Input: part model. Units: mm. Frame: model coordinates. A direction names the side the tool comes from. Give positions to 0.01 mm unless a question says otherwise; leave off trailing zeros. Order: outer loops, then holes, each group sorted by start corner. A loop starts at its lowest first (then second) coordinate and runs counter-clockwise, first axis right, second up. Notation, with made-up numbers: M 34.5,-34.5 L 78.5,-34.5 A22 ccw 78.5,0.5 Z; hole C 39.25,-28 d11. An arc over 180 degrees is marked long. Use a Markdown table: item, result.
from build123d import *

# Parameters (mm, degrees)
EXTRUDE_1_DEPTH     = 4
SKETCH_3_R          = 2
CUT_EXTRUDE_1_DEPTH = 272.02260581
SKETCH_4_R          = 10.5
SKETCH_4_R_2        = 1.5
CUT_EXTRUDE_2_DEPTH = 272.02260581
SKETCH_5_R          = 2
CUT_EXTRUDE_3_DEPTH = 272.02260581
SKETCH_6_W          = 10
SKETCH_6_H          = 62
CUT_EXTRUDE_4_DEPTH = 272.02260581
FILLET_1_R          = 10
SKETCH_7_W          = 13
SKETCH_7_H          = 13
CUT_EXTRUDE_5_DEPTH = 4
EXTRUDE_2_DEPTH     = 4
FILLET_2_R          = 10


with BuildPart() as part:
    # 草图2 → 凸台-拉伸1 (new body)
    with BuildSketch(Plane.XY):
        Polygon((0, 0), (-75, 0), (-75, -15), (-244.434557418, -15), (-55, -117), (0, -117), align=None)
    extrude(amount=EXTRUDE_1_DEPTH)

    # 草图3 → 切除-拉伸1 (cut, through all)
    with BuildSketch(Plane.XY.offset(4)):
        with Locations((-57.5, -6)):
            Circle(SKETCH_3_R)
        with Locations((-69, -17.5)):
            Circle(SKETCH_3_R)
        with Locations((-17.5, -6)):
            Circle(SKETCH_3_R)
        with Locations((-6, -17.5)):
            Circle(SKETCH_3_R)
        with Locations((-6, -57.5)):
            Circle(SKETCH_3_R)
        with Locations((-17.5, -69)):
            Circle(SKETCH_3_R)
        with Locations((-57.5, -69)):
            Circle(SKETCH_3_R)
        with Locations((-69, -57.5)):
            Circle(SKETCH_3_R)
    extrude(amount=-CUT_EXTRUDE_1_DEPTH, mode=Mode.SUBTRACT)

    # 草图4 → 切除-拉伸2 (cut, through all)
    with BuildSketch(Plane.XY.offset(4)):
        with Locations((-40, -100)):
            Circle(SKETCH_4_R)
        with Locations((-52.5, -112.5)):
            Circle(SKETCH_4_R_2)
        with Locations((-27.5, -112.5)):
            Circle(SKETCH_4_R_2)
        with Locations((-27.5, -87.5)):
            Circle(SKETCH_4_R_2)
        with Locations((-52.5, -87.5)):
            Circle(SKETCH_4_R_2)
    extrude(amount=-CUT_EXTRUDE_2_DEPTH, mode=Mode.SUBTRACT)

    # 草图5 → 切除-拉伸3 (cut, through all)
    with BuildSketch(Plane.XY.offset(4)):
        with Locations((-98.653292605, -71.825698472)):
            Circle(SKETCH_5_R)
        with Locations((-72.238972, -86.048344744)):
            Circle(SKETCH_5_R)
        with Locations((-160.286707351, -38.639523839)):
            Circle(SKETCH_5_R)
        with Locations((-186.701027956, -24.416877568)):
            Circle(SKETCH_5_R)
    extrude(amount=-CUT_EXTRUDE_3_DEPTH, mode=Mode.SUBTRACT)

    # 草图6 → 切除-拉伸4 (cut, through all)
    with BuildSketch(Plane.XY.offset(4)):
        with Locations((-5, -86)):
            Rectangle(SKETCH_6_W, SKETCH_6_H)
    extrude(amount=-CUT_EXTRUDE_4_DEPTH, mode=Mode.SUBTRACT)

    # 圆角1
    fillet_1_edges = [part.edges().sort_by_distance(p)[0] for p in [
        (0, -55, 2),
    ]]
    fillet(fillet_1_edges, radius=FILLET_1_R - 0.0001)  # a hair under: the kernel refuses the full size

    # 草图7 → 切除-拉伸5 (cut)
    with BuildSketch(Plane.XY.offset(4)):
        Polygon((-19.242640687, -15), (-55.757359313, -15), (-51.757359313, -19), (-23.242640687, -19), align=None)
        Polygon((-56, -23.242640687), (-60, -19.242640687), (-60, -55.757359313), (-56, -51.757359313), align=None)
        Polygon((-51.757359313, -56), (-55.757359313, -60), (-19.242640687, -60), (-23.242640687, -56), align=None)
        Polygon((-15, -55.757359313), (-15, -19.242640687), (-19, -23.242640687), (-19, -51.757359313), align=None)
        Polygon((-27.242640687, -23), (-47.757359313, -23), (-43.757359313, -27), (-31.242640687, -27), align=None)
        Polygon((-48, -31.242640687), (-52, -27.242640687), (-52, -47.757359313), (-48, -43.757359313), align=None)
        Polygon((-43.757359313, -48), (-47.757359313, -52), (-27.242640687, -52), (-31.242640687, -48), align=None)
        Polygon((-23, -47.757359313), (-23, -27.242640687), (-27, -31.242640687), (-27, -43.757359313), align=None)
        with Locations((-37.5, -37.5)):
            Rectangle(SKETCH_7_W, SKETCH_7_H)
    extrude(amount=-CUT_EXTRUDE_5_DEPTH, mode=Mode.SUBTRACT)

    # 草图8 → 凸台-拉伸2 (add)
    with BuildSketch(Plane.XY.offset(4)):
        with BuildLine():
            Line((-10, -117), (-55, -117))
            ThreePointArc((-55, -117), (-32.5, -122.672487724), (-10, -117))
        make_face()
    extrude(amount=-EXTRUDE_2_DEPTH)

    # 圆角2
    fillet_2_edges = [part.edges().sort_by_distance(p)[0] for p in [
        (-10, -117, 2),
        (-10, -55, 2),
        (-244.434557418, -15, 2),
        (-75, -15, 2),
    ]]
    fillet(fillet_2_edges, radius=FILLET_2_R)


solid = part.part
1) Reachability of faces 1 (the face through (-37, -56, 2)), 2 (the face through (-144, -15, 2)) from +Z, -Z, +X, -X, +Y, -Y: full face, straight path, thin tool, end or side. Return the list, or none.
Response values:
| item | result |
|---|---|
| face 1 | +Z, -Z |
| face 2 | +Z, -Z, -X, +Y |
2) First-contact query: pin 1 Ø5 at (x, y) = (-17.5, -6) entering from -Z; pin 2 Ø2 at (x, z) = (-37.5, 1) entering from -Y; pin 3 Ø1 at (x, z) = (-146.5, 3.5) entering from -Y; pin 4 Ø1.5 at (x, z) = (-133, 3.5) entering from -Y. Flat tips, straight axial feed; report the tip coordinate or a pass-through.
Response values:
| item | result |
|---|---|
| pin 1 | stops at z = 0 |
| pin 2 | stops at y = -122.5 |
| pin 3 | stops at y = -68 |
| pin 4 | stops at y = -75.41 |
3) Cut plane A-A on y = -100. Return loops of the section in (x, z).
Response values:
| item | result |
|---|---|
| outline | M -86.57,0 L -50.5,0 L -50.5,4 L -86.57,4 Z; M -29.5,0 L -10,0 L -10,4 L -29.5,4 Z |
4) Material intervals for line 1 (Y direction, x = -69, z = 1.9); line 2 (Y direction, x = -54.5, z = 2.3); line 3 (X direction, y = -112.5, z = 3.25), sorted ascending. Write a range as from..to.
Response values:
| item | result |
|---|---|
| line 1 | y = -109.46..-59.5, -55.5..-19.5, -15.5..0 |
| line 2 | y = -117.27..-60, -58.74..-16.26, -15..0 |
| line 3 | x = -63.36..-54, -51..-29, -26..-10.2 |
5) Cut plane D-D on y = -65. Return loops of the section in (x, z), and give its area (3 significant figures).
Response values:
| item | result |
|---|---|
| outline | M -151.57,0 L -10,0 L -10,4 L -151.57,4 Z |
| area | 566 mm² |
6) Cut plane B-B on x = -167. Return loops of the section in (y, z).
Response values:
| item | result |
|---|---|
| outline | M -56.69,0 L -15,0 L -15,4 L -56.69,4 Z |
7) Cut plane C-C on z = 2.95. State how many separate pieces and enclosed holes the cut face has, and give its area (3 significant figures).
Response values:
| item | result |
|---|---|
| separate pieces | 1 |
| enclosed holes | 25 |
| area | 14,200 mm² |
8) Mould query, pull axis X, two halves, no side actions, for faces 3 (the face through (-17.76, -67.017, 2.028)), 4 (the face through (-78.01, -12.15, 2.03)), 5 (the face through (-85, -47, 0)). Classes: released by +X, released by -X, zero draft, split by the parting line, or undercut.
Response values:
| item | result |
|---|---|
| face 3 | undercut |
| face 4 | released by -X |
| face 5 | zero draft |
